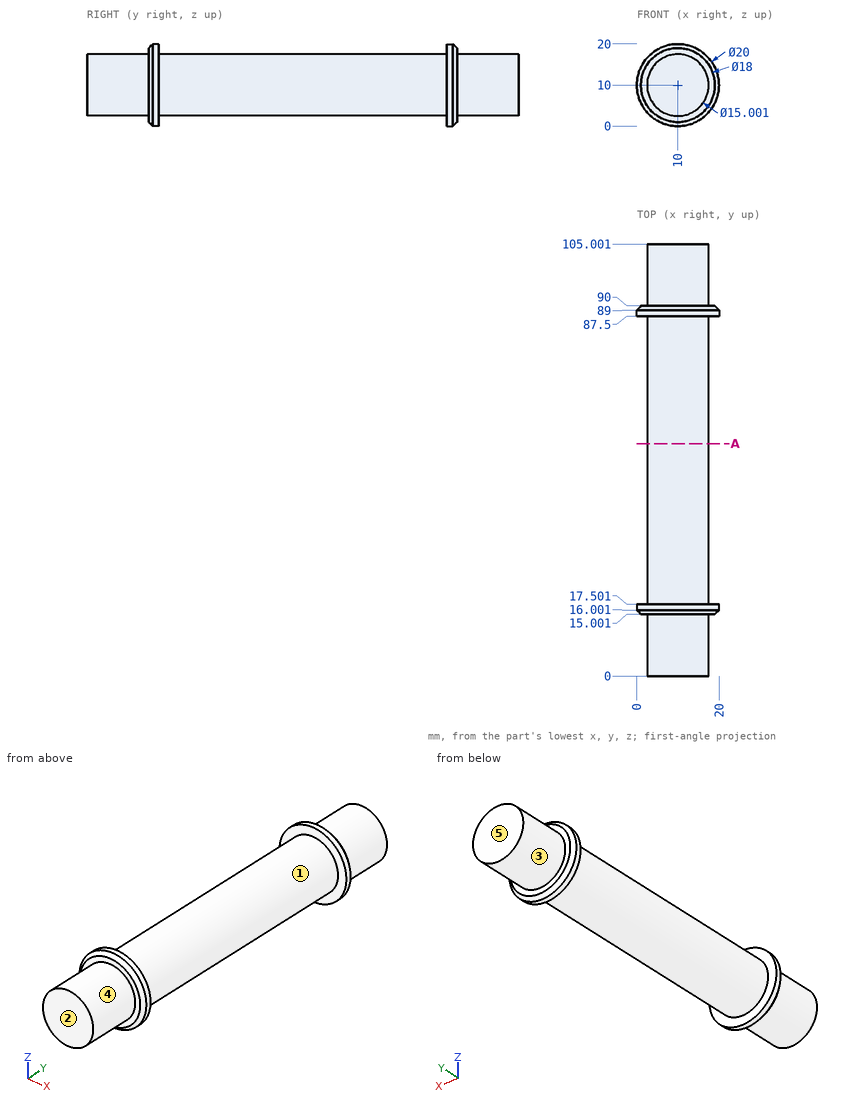
Job drawing, mm, ordinate dimensions from the low corner. One solid piece. A direction names the side the tool comes from. Round coordinates to 2 decimals unless told otherwise and drop trailing zeros. Loops run counter-clockwise (first coordinate to the right, second up) from the corner with the lowest first, then second, coordinate; pieces in that order, holes last.
Item 1: Drop flat-ended pins along their axis: P1, Ø10, axis at x = 17, y = 63.5, coming from the -Z side; P2, Ø9, axis at x = 13, z = 14.5, coming from the -Y side; P3, Ø2, axis at x = 9, y = 39, coming from the -Z side; P4, Ø4, axis at x = 16, y = 76.5, coming from the +Z side (1 decimal). Give the stop position or say it passes through.
Item 2: Mould opens along Y. For the marked faces 1, 2 and 3 say: +Y half, -Y half, draft (parallel to the pull), parting line (faces both ways), or undercut.
Item 3: Cut at A-A, the plane y = 56.5. Give the cut face in (x, z), then the cut area to 3 significant figures.
Item 4: 3-axis set-ups, long thin cutter, end or side, ignore diameter. For the marked faces 4 and 5: which of +Z, -Z, +X, -X, +Y, -Y reach the whole face in a straight line?
Item 5: Drill centre lines: line 1 (Y direction, x = 3, z = 5.25); line 2 (Z direction, x = 10.5, y = 61.5); line 3 (X direction, y = 14.5, z = 10.25). Where is each one in solid material? Low to high.
A:
1. P1: stops at z = 2.77
1. P2: stops at y = 0
1. P3: stops at z = 2.5
1. P4: stops at z = 16.3
2. face 1: undercut
2. face 2: -Y half
2. face 3: draft
3. outline: circle Ø15 at (10, 10)
3. area: 177 mm2
4. face 4: -Y
4. face 5: +Z, -Z, +X, -X, +Y
5. line 1: y = 15 to 17.5, 87.5 to 90
5. line 2: z = 2.52 to 17.48
5. line 3: x = 2.5 to 17.5
